Geometry: final body of the model. Coordinates: model frame, mm. A direction names the side the tool comes from. Give positions to 0.01 mm unless a question says otherwise; leave off trailing zeros. Write each loop counter-clockwise with the first axis right and the second up, starting at its lowest first coordinate (ties: lowest second). Pieces come first, ordered by that corner, then holes.
Q1. Cut plane B-B on x = 225. Return the cut outline in (y, z).
Q2. Pin query (flat end, axial travel): pin 1 (9 mm diameter, centred on y = 169.5, z = 5.5, fed in from -X); pin 2 (1.5 mm diameter, centred on x = 87, z = 9, fed in from +Y); pin 3 (9 mm diameter, centred on y = 61, z = 9, fed in from -X). Return the tip coordinate at first contact, or that it passes through.
Q3. Cut plane A-A on y = 39. Return the cut outline in (x, z).
Q4. Cut plane C-C on y = 0. Return the cut outline in (x, z).
Q5. Line query: L1, parallel to Y at x = -130.5, z = 1; L2, parallel to X at y = 171, z = 6.25; L3, parallel to Y at x = 225, z = 5.75. Output: solid intervals per line, ascending.
Q6. Reachability of faces 4 (the face through (67.739, 140, 9)), 5 (the face through (30, 178.43, 9)), 6 (the face through (-13.624, 85.129, 9.126)) from +Z, -Z, +X, -X, +Y, -Y: full face, straight path, thin tool, end or side. Return the list, or none.
Q7. Draft query along X for faces 1 (the face through (4, 27, 0)), 2 (the face through (-153.143, 85.21, 9.126)), 3 (the face through (236, 0, 9)). Return one class per face: pulls with the +X half, pulls with the -X half, needs draft (parallel to the pull), parting line crosses it, or undercut.
Q8. Cut plane D-D on z = 12. Return the cut outline in (x, y), plus the area to 3 significant figures.
```python
from build123d import *

# Parameters (mm, degrees)
SCHIZZO1_W                   = 600
SCHIZZO1_H                   = 100
ESTRUSIONE_ESTRUSIONE1_DEPTH = 18
SCHIZZO2_W                   = 400
SCHIZZO2_H                   = 18
TAGLIO_ESTRUSIONE1_DEPTH     = 18
SCHIZZO3_R                   = 11
TAGLIO_ESTRUSIONE2_DEPTH     = 18
SCHIZZO7_W                   = 111.74591768
SCHIZZO7_H                   = 50
ESTRUSIONE_ESTRUSIONE2_DEPTH = 18
SCHIZZO4_R                   = 11
TAGLIO_ESTRUSIONE4_DEPTH     = 18
SMUSSO1_SIZE                 = 30
SCHIZZO9_R                   = 4
ESTRUSIONE_ESTRUSIONE3_DEPTH = 18
ESTRUSIONE_ESTRUSIONE4_DEPTH = 18
SCHIZZO15_W                  = 19.88
SCHIZZO15_H                  = 19.28
TAGLIO_ESTRUSIONE7_DEPTH     = 20


with BuildPart() as part:
    # Schizzo1 → Estrusione-Estrusione1 (new body)
    with BuildSketch(Plane.XY):
        Rectangle(SCHIZZO1_W, SCHIZZO1_H)
    extrude(amount=ESTRUSIONE_ESTRUSIONE1_DEPTH)

    # Schizzo2 → Taglio-Estrusione1 (cut)
    with BuildSketch(Plane.XY.offset(18)):
        Rectangle(SCHIZZO2_W, SCHIZZO2_H)
    extrude(amount=-TAGLIO_ESTRUSIONE1_DEPTH, mode=Mode.SUBTRACT)

    # Schizzo3 → Taglio-Estrusione2 (cut)
    with BuildSketch(Plane.XY.offset(18)):
        with Locations((-225, 0)):
            Circle(SCHIZZO3_R)
    taglio_estrusione2 = extrude(amount=-TAGLIO_ESTRUSIONE2_DEPTH, mode=Mode.SUBTRACT)

    # Specchia1: Taglio-Estrusione2 across plane
    add(taglio_estrusione2.mirror(Plane(origin=(0, 0, 0), x_dir=(0, 0, 1), z_dir=(1, 0, 0))), mode=Mode.SUBTRACT)

    # Schizzo7 → Estrusione-Estrusione2 (add)
    with BuildSketch(Plane.XY.offset(18)):
        with Locations((-112.480128411, 75)):
            Rectangle(SCHIZZO7_W, SCHIZZO7_H)
    extrude(amount=-ESTRUSIONE_ESTRUSIONE2_DEPTH)

    # Schizzo4 → Taglio-Estrusione4 (cut)
    with BuildSketch(Plane.XY.offset(18)):
        with Locations((-112.480128411, 39)):
            Circle(SCHIZZO4_R)
    extrude(amount=-TAGLIO_ESTRUSIONE4_DEPTH, mode=Mode.SUBTRACT)

    # Smusso1
    smusso1_edges = [part.edges().sort_by_distance(p)[0] for p in [
        (-168.353087251, 100, 9),
        (-56.607169571, 100, 9),
    ]]
    chamfer(smusso1_edges, length=SMUSSO1_SIZE)

    # Schizzo9 → Estrusione-Estrusione3 (add)
    with BuildSketch(Plane.XY.offset(18)):
        Polygon((-1.816869292, 219.840422), (-1.816869292, 99.840422), (-41.816869292, 50), (78.183130708, 50), (67.739440982, 63.012947579), (67.739440982, 219.840422), align=None)
        with Locations((18.183130708, 199.840422)):
            Circle(SCHIZZO9_R, mode=Mode.SUBTRACT)
        with Locations((18.183130708, 134.750422)):
            Circle(SCHIZZO9_R, mode=Mode.SUBTRACT)
    extrude(amount=-ESTRUSIONE_ESTRUSIONE3_DEPTH)

    # Schizzo10 → Estrusione-Estrusione4 (add)
    with BuildSketch(Plane.XY.offset(18)):
        Polygon((-56.607169571, 70), (-25.765640833, 70), (-41.816869292, 50), (-56.607169571, 50), align=None)
    extrude(amount=-ESTRUSIONE_ESTRUSIONE4_DEPTH)

    # Schizzo15 → Taglio-Estrusione7 (cut)
    with BuildSketch(Plane.XY.offset(18)):
        with Locations((30.563130708, 168.790422)):
            Rectangle(SCHIZZO15_W, SCHIZZO15_H)
    extrude(amount=-TAGLIO_ESTRUSIONE7_DEPTH, mode=Mode.SUBTRACT)


solid = part.part
```
Data:
1. outline: (-50, 0) - (-11, 0) - (-11, 18) - (-50, 18) - close; (11, 0) - (50, 0) - (50, 18) - (11, 18) - close
2. pin 1: stops at x = -1.82
2. pin 2: stops at y = 50
2. pin 3: stops at x = -168.35
3. outline: (-300, 0) - (-123.48, 0) - (-123.48, 18) - (-300, 18) - close; (-101.48, 0) - (300, 0) - (300, 18) - (-101.48, 18) - close
4. outline: (-300, 0) - (-236, 0) - (-236, 18) - (-300, 18) - close; (-214, 0) - (-200, 0) - (-200, 18) - (-214, 18) - close; (200, 0) - (214, 0) - (214, 18) - (200, 18) - close; (236, 0) - (300, 0) - (300, 18) - (236, 18) - close
5. L1: y = -50 to -9, 9 to 100
5. L2: x = -1.82 to 20.62, 40.5 to 67.74
5. L3: y = -50 to -11, 11 to 50
6. face 4: +Z, -Z, +X, +Y
6. face 5: +Z, -Z
6. face 6: +Z, -Z, +Y
7. face 1: needs draft
7. face 2: pulls with the -X half
7. face 3: undercut
8. outline: (-300, -50) - (300, -50) - (300, 50) - (78.18, 50) - (67.74, 63.01) - (67.74, 219.84) - (-1.82, 219.84) - (-1.82, 99.84) - (-25.77, 70) - (-56.61, 70) - (-86.61, 100) - (-138.35, 100) - (-168.35, 70) - (-168.35, 50) - (-300, 50) - close; hole circle Ø22 at (-225, 0); hole (-200, -9) - (200, -9) - (200, 9) - (-200, 9) - close; hole circle Ø22 at (-112.48, 39); hole circle Ø8 at (18.18, 134.75); hole circle Ø8 at (18.18, 199.84); hole (20.62, 159.15) - (40.5, 159.15) - (40.5, 178.43) - (20.62, 178.43) - close; hole circle Ø22 at (225, 0)
8. area: 69,200 mm2
